Source: CAD feature listing. Evaluate the final solid. Frame: model axes, mm. Face numbers are marked on the shaded views. A direction names the side the tool comes from. Coordinates: 2 decimals unless noted, no trailing zeros. Order: outer loops, then holes, each group sorted by start corner. A loop starts at its lowest first (then second) coordinate and runs counter-clockwise, first axis right, second up. Notation, with made-up numbers: (63, 43.25) -> (74, 43.25) arc R15 cw to (74, 67.25) -> close; hole circle Ø11 at (46, 16). An arc over 180 degrees is marked (long way). Put each result on its own line as item: value.
from build123d import *

# Parameters (mm, degrees)
F0_W     = 203.2
F0_H     = 127
F1_DEPTH = 127
F3_DEPTH = 76.2
F4_SIZE2 = 76.2
F4_SIZE  = 50.8
F5_R     = 5.08
F6_R     = 15.24
F7_DEPTH = 50.8


with BuildPart() as f1:
    # F0 (on Front) → F1 (new body)
    with BuildSketch(Plane.XZ):
        Rectangle(F0_W, F0_H)
    extrude(amount=F1_DEPTH)

    # F2 (on face) → F3 (cut)
    with BuildSketch(Plane.XZ.offset(127)):
        Polygon((101.6, 63.5), (0, 63.5), (0, 0), (-50.8, 0), (-50.8, -63.5), (101.6, -63.5), align=None)
    extrude(amount=-F3_DEPTH, mode=Mode.SUBTRACT)

    # F4
    f4_edges = [f1.edges().sort_by_distance(p)[0] for p in [
        (101.6, -25.4, 63.5),
    ]]
    f4_side = f1.faces().sort_by_distance((-21.771429, -52.614286, 63.5))[0]
    chamfer(f4_edges, length=F4_SIZE, length2=F4_SIZE2, reference=f4_side)

    # F5
    f5_edges = [f1.edges().sort_by_distance(p)[0] for p in [
        (25.4, -50.8, 63.5),
        (-25.4, 0, 63.5),
        (50.8, -25.4, 63.5),
        (-101.6, -63.5, 63.5),
        (-50.8, -127, 63.5),
        (0, -88.9, 63.5),
        (0, -127, 31.75),
        (0, -50.8, 31.75),
        (-50.8, -88.9, -63.5),
        (25.4, -50.8, -63.5),
        (-50.8, -50.8, -31.75),
        (-50.8, -127, -31.75),
        (-25.4, -127, 0),
        (-101.6, -127, 0),
    ]]
    fillet(f5_edges, radius=F5_R)

    # F6 (on face) → F7 (cut, through all)
    with BuildSketch(Plane.XZ.offset(50.8)):
        with Locations((5.08, -17.78)):
            Circle(F6_R)
    extrude(amount=-F7_DEPTH, mode=Mode.SUBTRACT)


solid = f1.part
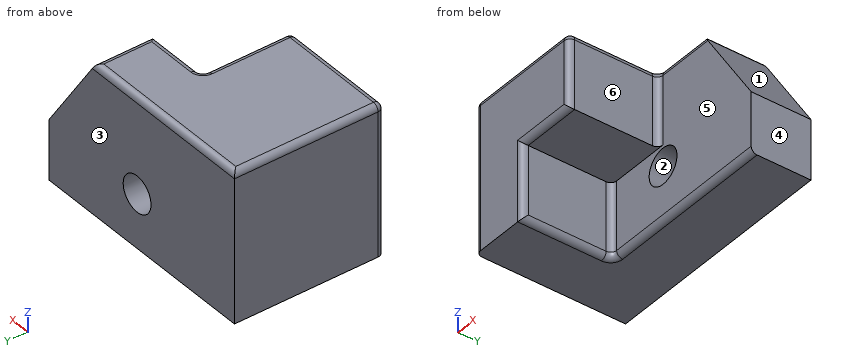
1. Cut plane D-D on x = -43.5. Output: boundary loops of the cut face in (y, z), plus the area to 3 significant figures.
Numbers:
outline: (-127, 5.08) arc R5.08 ccw to (-121.92, 0) -> (-50.8, 0) -> (-50.8, -58.42) arc R5.08 ccw to (-45.72, -63.5) -> (0, -63.5) -> (0, 58.42) arc R5.08 ccw to (-5.08, 63.5) -> (-121.92, 63.5) arc R5.08 ccw to (-127, 58.42) -> close
area: 11,300 mm2
2. Pull-direction query (X, two-part tool) for the marked faces 1, 2 and 3; classes: pulls with the +X half, pulls with the -X half, needs draft (parallel to the pull), parting line crosses it, or undercut.
Numbers:
face 1: pulls with the +X half
face 2: undercut
face 3: needs draft
3. Set-up query: the marked faces 4, 5 and 6. Return all of +Z, -Z, +X, -X, +Y, -Y with unobstructed straight access to the full face (end or side cutting, diameter ignored); none if empty.
Numbers:
face 4: +Z, -Z, +X, +Y, -Y
face 5: -Z, +X, -Y
face 6: +Z, -Z, +X, -Y
4. First-contact query: pin 1 (6 mm diameter, centred on y = -70, z = 11, fed in from +X); pin 2 (1 mm diameter, centred on y = -94.5, z = -49.5, fed in from +X); pin 3 (5 mm diameter, centred on y = -34.5, z = 47, fed in from +X). Flat tips, straight axial feed; report the tip coordinate or a pass-through.
Numbers:
pin 1: stops at x = 0
pin 2: stops at x = -50.8
pin 3: stops at x = 63.47
5. Cut plane C-C on y = -111. Output: boundary loops of the cut face in (x, z).
Numbers:
outline: (-101.6, -63.5) -> (-55.88, -63.5) arc R5.08 ccw to (-50.8, -58.42) -> (-50.8, 0) -> (0, 0) -> (0, 58.42) arc R5.08 ccw to (-5.08, 63.5) -> (-96.52, 63.5) arc R5.08 ccw to (-101.6, 58.42) -> close
6. Cut plane A-A on y = -23. Output: boundary loops of the cut face in (x, z).
Numbers:
outline: (-101.6, -63.5) -> (101.6, -63.5) -> (101.6, -12.7) -> (52.31, 61.24) arc R5.08 ccw to (48.08, 63.5) -> (-96.52, 63.5) arc R5.08 ccw to (-101.6, 58.42) -> close; hole circle Ø30.48 at (5.08, -17.78)
7. Cut plane B-B on z = -17.78. Output: boundary loops of the cut face in (x, y), plus the area to 3 significant figures.
Numbers:
outline: (-101.6, -121.92) arc R5.08 ccw to (-96.52, -127) -> (-55.88, -127) arc R5.08 ccw to (-50.8, -121.92) -> (-50.8, -55.88) arc R5.08 cw to (-45.72, -50.8) -> (-10.16, -50.8) -> (-10.16, 0) -> (-101.6, 0) -> close; (20.32, -50.8) -> (101.6, -50.8) -> (101.6, 0) -> (20.32, 0) -> close
area: 12,600 mm2
8. Ray query, line 1 along Z through (x, y) = (5, -17); line 2 along X through (y, z) = (-32, -17); line 3 along Z through (x, y) = (-49.5, -69). Return the intervals inside material, ascending.
Numbers:
line 1: z = -63.5 to -33.02, -2.54 to 63.5
line 2: x = -101.6 to -10.14, 20.3 to 101.6
line 3: z = 0 to 63.5
